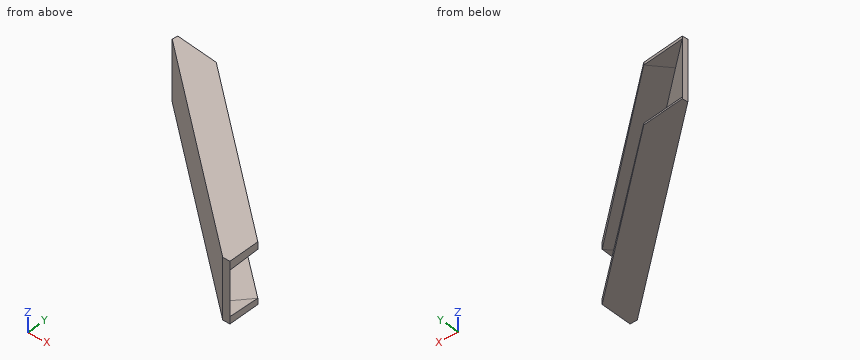
Autodesk Inventor part; units mm, degrees
ref_plane "Work Plane1" through (-511.6606, -738.8097, -32.3222) normal (-0.6447648, -0.764381, 0) x (0.764381, -0.6447648, 0)
ref_plane "YZ Plane" through (0, 0, 0) normal (1, 0, 0) x (0, 1, 0)
ref_plane "XZ Plane" through (0, 0, 0) normal (0, 1, 0) x (-1, 0, 0)
sketch "Sketch1" plane through (0, 0, 0) normal (0, 0, 1) x (1, 0, 0)
  line L0 (-381.58, -848.5343) -> (-381.58, -825.2737)
  line L1 (-381.58, -825.2737) -> (-505.1463, -721.0439)
  line L2 (-505.1463, -721.0439) -> (-536.6679, -717.7157)
  line L3 (-381.58, -848.5343) -> (-386.946, -848.5205)
  line L4 (-386.946, -848.5205) -> (-537.1054, -721.8591)
  line L5 (-537.1054, -721.8591) -> (-536.6679, -717.7157)
  line L6 (-381.58, -848.5343) -> (-536.6679, -717.7157) construction
  point P0 (0, 0)
extrude "Extrusion1" add sketch "Sketch1" along normal mid plane 44.45
sketch "Sketch2" plane through (-505.1463, -721.0439, 22.225) normal (0.6447648, 0.764381, 0) x (0.764381, -0.6447648, 0)
  line L0 (0, 1.9422) -> (161.6554, 5.3274)
  line L1 (161.6554, 40.0134) -> (0, 43.18)
  line L2 (161.6554, 5.3274) -> (176.6531, 6.2699)
  line L3 (176.6531, 39.2056) -> (161.6554, 40.0134)
  line L4 (-26.2404, 2.0211) -> (0, 1.9422)
  line L5 (-26.2404, 43.18) -> (0, 43.18)
  line L6 (176.6531, 6.2699) -> (176.6531, 39.2056)
  line L7 (176.6531, 44.45) -> (176.6531, 0)
  line L8 (-26.2404, 2.0211) -> (-26.2404, 43.18)
  point P0 (-78.7795, 22.225)
ref_plane "Work Plane1" through (-511.6606, -738.8097, -32.3222) normal (-0.6447648, -0.764381, 0) x (0.764381, -0.6447648, 0)
extrude "Extrusion2" cut sketch "Sketch2" against normal up to surface (17.78 mm away)
properties part number "TopGrip"
Source: CAD feature listing. Evaluate the final solid. Frame: model axes, mm. Give positions to 0.01 mm unless a question says otherwise; leave off trailing zeros. Write each loop counter-clockwise with the first axis right and the second up, starting at its lowest first coordinate (ties: lowest second). Pieces come first, ordered by that corner, then holes. Notation, with made-up numbers: M 28,34.25 L 48,34.25 A25 cw 48,46.25 Z; hole C 62,55 d9. An arc over 180 degrees is marked long. Return JSON: item names as keys, results as strings. Group by question number.
1) Cut plane B-B, the plane y = -792.5. Output: boundary loops of the cut face in (x, z) (3 decimals).
2) First-contact query: pin 1 Ø3 at (x, z) = (-401.5, 6.5) entering from +Y; pin 2 Ø8 at (x, z) = (-509.5, 10.5) entering from -Y; pin 3 Ø3 at (x, z) = (-508, -16) entering from -Y. Flat tips, straight axial feed; report the tip coordinate or a pass-through.
3) Ray query, L1, parallel to Z at x = -474.5, y = -759.5 (3 decimals); L2, parallel to X at y = -801.5, z = 5; L3, parallel to X at y = -746, z = 19. Return the intervals inside material, ascending.
4) Cut plane C-C, the plane z = -3. Output: boundary loops of the cut face in (x, y).
5) Cut plane A-A, the plane x = -439. Output: boundary loops of the cut face in (y, z) (3 decimals), then the cut area to 3 significant figures.
Data:
{
 "1": {"outline": "M -453.359,-22.225 L -420.434,-22.225 L -420.434,-18.784 L -448.013,-19.197 L -448.013,18.403 L -420.434,17.962 L -420.434,22.225 L -453.359,22.225 Z"},
 "2": {"pin 1": "stops at y = -830.47", "pin 2": "stops at y = -748.52", "pin 3": "stops at y = -747.68"},
 "3": {"L1": "z = -22.225 to -20.01, 19.273 to 22.225", "L2": "x = -442.69 to -437.34", "L3": "x = -508.49 to -503.14"},
 "4": {"outline": "M -537.11,-721.86 L -386.95,-848.52 L -381.58,-848.53 L -536.67,-717.72 Z"},
 "5": {"outline": "M -804.612,-22.225 L -776.839,-22.225 L -776.839,-19.26 L -800.102,-18.966 L -800.102,18.157 L -776.839,18.471 L -776.839,22.225 L -804.612,22.225 Z", "area": "364 mm²"}
}
